Model file for the job. Use its own axes, mm. Face numbers are marked on the shaded views. A direction names the side the tool comes from. Give positions to 0.01 mm unless a question says otherwise; leave off trailing zeros. Loops run counter-clockwise (first coordinate to the right, second up) from the corner with the lowest first, then second, coordinate; pieces in that order, holes last. Notation, with made-up numbers: (47.5, 9) - (88.5, 9) arc R17 cw to (88.5, 24) - close; hole circle Ø8 at (65.25, 43.25). An arc over 180 degrees is marked (long way). Use a Markdown table: item, result.
from build123d import *

# Parameters (mm, degrees)
ESBO_O4_W                           = 5.9436
ESBO_O4_H                           = 29.356
FURO_ROSCADO_DE_1_4_18_NPSM3_REACH  = 70.621
FURO_ROSCADO_DE_1_4_18_NPSM3_BORE_R = 5.9436
ESBO_O12_R                          = 16
ESBO_O12_R_2                        = 9
RESSALTO_EXTRUS_O1_DEPTH            = 1
PADR_OCIRCULAR5_COUNT               = 4
CHANFRO1_SIZE                       = 0.5
CHANFRO2_SIZE                       = 0.25
FURO_ROSCADO_DE_1_4_18_NPSM2_D      = 11.8872
ESBO_O18_R                          = 8.5
CORTE_EXTRUS_O4_DEPTH               = 1.5
ESBO_O20_R                          = 8.5
CORTE_EXTRUS_O5_DEPTH               = 1.5
CORTE_EXTRUS_O6_DEPTH               = 54.033475186


with BuildPart() as part:
    # Esboço1 → Revolução1 (revolve)
    with BuildSketch(Plane.XY, mode=Mode.PRIVATE) as revolu_o1_sk:
        Polygon((0, -20), (29.356, -20), (29.356, 13), (9, 13), (9, -13), (3, -13), (3, -17.6), (0, -17.6), align=None)
    revolve(revolu_o1_sk.sketch.rotate(Axis((0, -20, 0), (0, 1, 0)), 90), axis=Axis((0, -20, 0), (0, 1, 0)))

    # Esboço4 → Furo roscado de 1/4-18 NPSM1 (revolve, cut)
    with BuildSketch(Plane(origin=(29.356, 0, 0), x_dir=(0, 0, -1), z_dir=(0, 1, 0))):
        with Locations((2.9718, 14.678)):
            Rectangle(ESBO_O4_W, ESBO_O4_H)
    revolve(axis=Axis((35.706, 0, 0), (-1, 0, 0)), mode=Mode.SUBTRACT)

    # Furo roscado de 1/4-18 NPSM3 bore → Furo roscado de 1/4-18 NPSM3 (cut, up to next)
    with BuildSketch(Plane(origin=(0, 0, -29.356), x_dir=(0, -1, 0), z_dir=(0, 0, -1)), mode=Mode.PRIVATE) as furo_roscado_de_1_4_18_npsm3_sk1:
        Circle(FURO_ROSCADO_DE_1_4_18_NPSM3_BORE_R)
    furo_roscado_de_1_4_18_npsm3_tool1 = extrude(furo_roscado_de_1_4_18_npsm3_sk1.sketch, amount=-FURO_ROSCADO_DE_1_4_18_NPSM3_REACH, mode=Mode.PRIVATE) & part.part
    add(furo_roscado_de_1_4_18_npsm3_tool1.solids().sort_by_distance((0, 0, -29.356))[0], mode=Mode.SUBTRACT)

    # Esboço12 → Ressalto-extrusão1 (add)
    with BuildSketch(Plane(origin=(0, 13, 0), x_dir=(1, 0, 0), z_dir=(0, 1, 0))):
        with Locations(Location((0, 0, 0), (0, 0, 270))):
            Circle(ESBO_O12_R)
        with Locations(Location((0, 0, 0), (0, 0, 90))):
            Circle(ESBO_O12_R_2, mode=Mode.SUBTRACT)
    extrude(amount=RESSALTO_EXTRUS_O1_DEPTH)

    # Esboço13 → Furo roscado de M3x0.51 (revolve, cut)
    with BuildSketch(Plane(origin=(8.838834765, 14, -8.838834765), x_dir=(0, 0, 1), z_dir=(1, 0, 0))):
        Polygon((0, 0), (0, 10.751075774), (1.25, 10), (1.25, 0), align=None)
    furo_roscado_de_m3x0_51 = revolve(axis=Axis((8.838834765, 20.35, -8.838834765), (0, -1, 0)), mode=Mode.SUBTRACT)

    # PadrãoCircular5: Furo roscado de M3x0.51 ×4 about axis
    padr_ocircular5_axis = Axis((0, 0, 0), (0, 1, 0))
    for i in range(1, PADR_OCIRCULAR5_COUNT):
        add(furo_roscado_de_m3x0_51.rotate(padr_ocircular5_axis, i * 360 / PADR_OCIRCULAR5_COUNT), mode=Mode.SUBTRACT)

    # Chanfro1
    chanfro1_edges = [part.edges().sort_by_distance(p)[0] for p in [
        (0, -13, 3),
    ]]
    chamfer(chanfro1_edges, length=CHANFRO1_SIZE)

    # Chanfro2
    chanfro2_edges = [part.edges().sort_by_distance(p)[0] for p in [
        (0, 14, 9),
    ]]
    chamfer(chanfro2_edges, length=CHANFRO2_SIZE)

    # Furo roscado de 1/4-18 NPSM2 (through all)
    with Locations(Plane(origin=(-29.356, 0, 0), x_dir=(0, 0, -1), z_dir=(-1, 0, 0))):
        with Locations((0, 0)):
            Hole(FURO_ROSCADO_DE_1_4_18_NPSM2_D / 2)

    # Esboço18 → Corte-extrusão4 (cut)
    with BuildSketch(Plane(origin=(-29.356, 0, 0), x_dir=(0, -1, 0), z_dir=(-1, 0, 0))):
        with Locations(Location((0, 0, 0), (0, 0, 90))):
            Circle(ESBO_O18_R)
    corte_extrus_o4 = extrude(amount=-CORTE_EXTRUS_O4_DEPTH, mode=Mode.SUBTRACT)

    # Esboço20 → Corte-extrusão5 (cut)
    with BuildSketch(Plane(origin=(0, 0, -29.356), x_dir=(0, -1, 0), z_dir=(0, 0, 1))):
        Circle(ESBO_O20_R)
    extrude(amount=CORTE_EXTRUS_O5_DEPTH, mode=Mode.SUBTRACT)

    # Espelhar1: Corte-extrusão4 across plane
    add(corte_extrus_o4.mirror(Plane(origin=(0, 0, 0), x_dir=(0, 0, 1), z_dir=(1, 0, 0))), mode=Mode.SUBTRACT)

    # Esboço21 → Corte-extrusão6 (cut, through all)
    with BuildSketch(Plane(origin=(0, 13, 0), x_dir=(1, 0, 0), z_dir=(0, 1, 0))):
        with BuildLine():
            Line((-23.189970591, -18), (23.189970591, -18))
            ThreePointArc((23.189970591, -18), (0, -29.356), (-23.189970591, -18))
        make_face()
    extrude(amount=-CORTE_EXTRUS_O6_DEPTH, mode=Mode.SUBTRACT)


solid = part.part
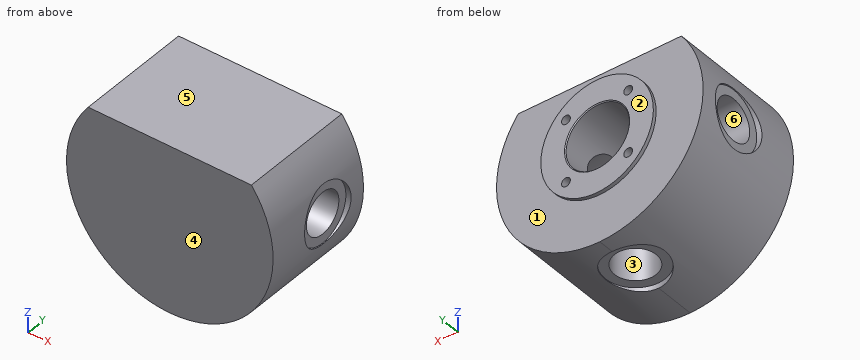
(1) Mould opens along Y. For the marked faces 4, 5 and 6 say: pulls with the +Y half, pulls with the -Y half, needs draft (parallel to the pull), parting line crosses it, or undercut.
Computed:
| item | result |
|---|---|
| face 4 | pulls with the -Y half |
| face 5 | needs draft |
| face 6 | undercut |
(2) Slice it at D-D, the plane y = 11. Write the cut outline in (x, z).
Computed:
| item | result |
|---|---|
| outline | (-23.19, 18) arc R29.36 ccw (long way) to (23.19, 18) - close; hole circle Ø2.5 at (-8.84, -8.84); hole circle Ø2.5 at (-8.84, 8.84); hole circle Ø18 at (0, 0); hole circle Ø2.5 at (8.84, -8.84); hole circle Ø2.5 at (8.84, 8.84) |
(3) 3-axis set-ups, long thin cutter, end or side, ignore diameter. For the marked faces 1, 2 and 3: which of +Z, -Z, +X, -X, +Y, -Y reach the whole face in a straight line?
Computed:
| item | result |
|---|---|
| face 1 | +Y |
| face 2 | +Z, -Z, +X, -X, +Y |
| face 3 | -Z |
(4) Slice it at A-A, the plane y = 0. Write the cut outline in (x, z), plus the area to 3 significant figures.
Computed:
| item | result |
|---|---|
| outline | (-28.1, -8.5) arc R29.36 ccw to (-8.5, -28.1) - (-8.5, -27.86) - (-5.94, -27.86) - (-5.94, -6.76) arc R9 cw to (-6.76, -5.94) - (-27.86, -5.94) - (-27.86, -8.5) - close; (-28.1, 8.5) - (-27.86, 8.5) - (-27.86, 5.94) - (-6.76, 5.94) arc R9 cw to (6.76, 5.94) - (27.86, 5.94) - (27.86, 8.5) - (28.1, 8.5) arc R29.36 ccw to (23.19, 18) - (-23.19, 18) arc R29.36 ccw to start; (5.94, -27.86) - (8.5, -27.86) - (8.5, -28.1) arc R29.36 ccw to (28.1, -8.5) - (27.86, -8.5) - (27.86, -5.94) - (6.76, -5.94) arc R9 cw to (5.94, -6.76) - close |
| area | 1,330 mm² |
(5) Slice it at C-C, the plane x = -11. Write the cut outline in (y, z), plus the area to 3 significant figures.
Computed:
| item | result |
|---|---|
| outline | (-20, -27.22) - (13, -27.22) - (13, -11.62) - (14, -11.62) - (14, 11.62) - (13, 11.62) - (13, 18) - (-20, 18) - close; hole circle Ø11.89 at (0, 0) |
| area | 1,400 mm² |
(6) Slice it at B-B, the plane z = 0. Count the separate pieces of the cut face and the enclosed holes in it, plus the area to 3 significant figures.
Computed:
| item | result |
|---|---|
| separate pieces | 3 |
| enclosed holes | 0 |
| area | 956 mm² |
(7) Pin check, flat tips, straight feed: P1, Ø5.5, axis at x = -4.5, z = 4, coming from the +Y side; P2, Ø8, axis at x = 5, y = 1, coming from the -Z side; P3, Ø2, axis at x = 9.5, y = -15.5, coming from the -Z side; P4, Ø3, axis at x = -8.84, z = 8.84, coming from the +Y side. Stop position of each tip, or through.
Computed:
| item | result |
|---|---|
| P1 | y = -13 |
| P2 | z = -28.41 |
| P3 | z = -28.1 |
| P4 | y = 14 |
(8) Drill centre lines: probe 1 along Z at (x, y) = (0, 7.75); probe 2 along Y at (x, z) = (28.2, 0); probe 3 along Y at (x, z) = (-16, 10.5). Where is each one in solid material? Low to high. Write a range as [from, to].
Computed:
| item | result |
|---|---|
| probe 1 | [-27.86, -9], [9, 18] |
| probe 2 | [-20, -8.5], [8.5, 13] |
| probe 3 | [-20, 13] |
